from build123d import *

# Parameters (mm, degrees)
F0_W        = 12.7
F0_H        = 8.8700183392
F0_H_2      = 25.4
F2_DEPTH    = 2.54
F3_DEPTH    = 2.54
F4_R        = 2.53999
F5_T1_DEPTH = 76.5737284666
F6_T1_DEPTH = 62.0182579324


# Not quite as in the source:
# - a fillet or chamfer that OpenCascade refuses, or shapes differently, is made with other operations: its cross-section is extruded or revolved along the edge and cut away or added
# - a fillet or chamfer is up to 0.001 mm smaller than in the source, because OpenCascade refuses the exact size


with BuildPart() as f2:
    # F0 (on Front) → F2 (new body, symmetric)
    with BuildSketch(Plane.XZ):
        with Locations((-23.8077666163, 5.7760581046)):
            Rectangle(F0_W, F0_H)
        with Locations((-23.8077666163, -11.3589510649)):
            Rectangle(F0_W, F0_H_2)
        with Locations((-36.5077666163, 5.7760581046)):
            Rectangle(F0_W, F0_H)
        with Locations((-11.1077666163, 5.7760581046)):
            Rectangle(F0_W, F0_H)
    extrude(amount=F2_DEPTH, both=True)

    # F1 (on Front) → F3 (join, symmetric)
    with BuildSketch(Plane.XZ):
        Polygon((-30.3534455597, 10.2110672742), (-17.4847040325, 10.2110672742), (-17.4847040325, 55.5314160883), (-23.9190747961, 64.7633413825), (-30.3534455597, 55.5314160883), align=None)
    extrude(amount=F3_DEPTH, both=True)

    # F4 (radius 2.54 in the source; OpenCascade refuses exactly that, so slightly less here)
    f4_edges = [f2.edges().sort_by_distance(p)[0] for p in [
        (-11.107767, 2.54, 1.341049),
        (-11.107767, -2.54, 1.341049),
        (-11.121235, 2.54, 10.211067),
        (-11.121235, -2.54, 10.211067),
        (-4.757767, -2.54, 5.776058),
        (-4.757767, 2.54, 5.776058),
        (-4.757767, 0, 10.211067),
        (-4.757767, 0, 1.341049),
        (-36.605606, -2.54, 10.211067),
        (-36.605606, 2.54, 10.211067),
        (-36.507767, -2.54, 1.341049),
        (-36.507767, 2.54, 1.341049),
        (-42.857767, -2.54, 5.776058),
        (-42.857767, 2.54, 5.776058),
        (-42.857767, 0, 10.211067),
        (-17.457767, 2.54, -11.358951),
        (-17.457767, -2.54, -11.358951),
        (-30.157767, -2.54, -11.358951),
        (-30.157767, 2.54, -11.358951),
        (-23.807767, -2.54, -24.058951),
        (-30.157767, 0, -24.058951),
        (-23.807767, 2.54, -24.058951),
        (-17.457767, 0, -24.058951),
    ]]
    fillet(f4_edges, radius=F4_R)

    # F5: chamfer of 12.7 on 1 edges, made by hand

    # F5_s2 → F5_t1 (cut)
    with BuildSketch(Plane(origin=(-13.0912626788, 0, 18.7831201367), x_dir=(0, 1, 0), z_dir=(-0.5717925773, 0, 0.8203982256))):
        Polygon((2.54, -4.7080313623), (-10.16, -17.4080313623), (2.54, -17.4080313623), align=None)
    extrude(amount=F5_T1_DEPTH, mode=Mode.SUBTRACT)

    # F6: chamfer of 7.62 on 1 edges, made by hand

    # F6_s2 → F6_t1 (cut)
    with BuildSketch(Plane(origin=(-10.0507456007, 0, 14.4206381549), x_dir=(0, 1, 0), z_dir=(-0.5717925773, 0, 0.8203982256))):
        Polygon((-2.8481536726, -10.0961850349), (2.54, 2.9119686377), (2.54, -4.7080313623), align=None)
    extrude(amount=F6_T1_DEPTH, mode=Mode.SUBTRACT)


solid = f2.part
Work out the finished part from the listing and answer in its coordinate system (mm). A direction names the side the tool comes from. Coordinates: 2 decimals unless noted, no trailing zeros. Loops run counter-clockwise (first coordinate to the right, second up) from the corner with the lowest first, then second, coordinate; pieces in that order, holes last. Notation, with made-up numbers: M 5.25,-10 L 51.25,-10 A28 ccw 51.25,9 Z; hole C 50.25,-16 d5. An arc over 180 degrees is marked long. Answer in a Markdown table with one row per item. Add a question column.
1. Flat-ended cylindrical pins translate along their axes: P1, Ø1, axis at y = -1, z = 28, coming from the +X side; P2, Ø1, axis at x = -14, y = 1.5, coming from the -Z side; P3, Ø1.5, axis at y = 0.5, z = 29, coming from the -X side. Find the tip coordinate at first contact, or state that the pin passes through.
2. Consider L1, parallel to X at y = -1.3, z = 18; L2, parallel to Z at x = -39.5, y = -0.5; L3, parallel to X at y = -0.5, z = 8.5. Determine where each line is inside the solid, lowest interval first.
3. Find section C-C, the plane z = 36. Write down the section's boundary in (x, y), then the cut area to 3 significant figures.
4. A tool of negligible diameter and unlimited length cuts with its end or side. For faces 1 (the cylindrical face through (-18.222, 1.816, -8.641)), 2 (the cylindrical face through (-12.463, -1.816, 9.447)), 3 (the cylindrical face through (-29.43, 1.78, -9)), 4 (the cylindrical face through (-35.405, 1.816, 9.447)), 5 (the cylindrical face through (-35.131, -1.816, 2.105)), from which of +Z, -Z, +X, -X, +Y, -Y can it reach the whole face along a straight path? Write none if from no direction.
Reported:
| question | item | result |
|---|---|---|
| 1 | P1 | stops at x = -17.48 |
| 1 | P2 | stops at z = 1.55 |
| 1 | P3 | stops at x = -30.35 |
| 2 | L1 | x = -30.35 to -17.48 |
| 2 | L2 | z = 1.39 to 10.16 |
| 2 | L3 | x = -42.67 to -4.95 |
| 3 | outline | M -30.35,-2.54 L -17.48,-2.54 L -17.48,-1.25 L -28.64,2.54 L -30.35,2.54 Z |
| 3 | area | 44.2 mm^2 |
| 4 | face 1 | -Z, +X, +Y |
| 4 | face 2 | +Z, +X, -Y |
| 4 | face 3 | -Z, -X, +Y |
| 4 | face 4 | +Z, -X, +Y |
| 4 | face 5 | -Z, -X, -Y |
